Could you check a few things on this model? Use its own coordinates, in mm. Face numbers are marked on the shaded views. A direction names the side the tool comes from. Give positions to 0.01 mm unless a question says otherwise; leave off trailing zeros. Write each loop counter-clockwise with the first axis right and the second up, starting at its lowest first coordinate (ties: lowest second). Pieces come first, ordered by that corner, then holes. Notation, with made-up numbers: M 41.25,58 L 57.25,58 A17 ccw 57.25,66 Z; hole C -36.5,42 d5. An arc over 180 degrees is marked long. Answer as a JSON object with one key per item and string values. Group by question number.
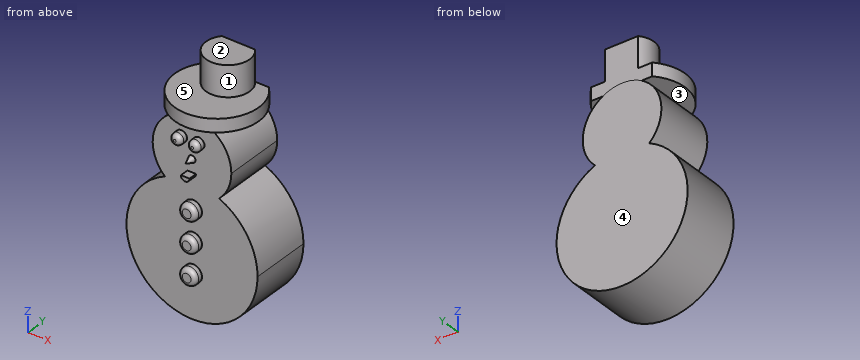
```python
from build123d import *

# Parameters (mm, degrees)
F1_DEPTH  = 7
F2_DEPTH  = 7
F3_R      = 1
F4_DEPTH  = 1
F5_DEPTH  = 1
F6_DEPTH  = 1
F7_R      = 0.65
F8_DEPTH  = 1
F9_DEPTH  = 1
F14_DEPTH = 1.5
F16_DEPTH = 3.5
F18_DEPTH = 1
F19_R     = 0.5


# Not quite as in the source:
# - a feature names something its author has since deleted; it is built from what else it names


with BuildPart() as f1:
    # F0 (on Front) → F1 (new body)
    with BuildSketch(Plane.XZ):
        with BuildLine():
            ThreePointArc((-3.1083265336, 6.8255626992), (0, 5.5795304558), (3.1083265336, 6.8255626992))
            ThreePointArc((3.1083265336, 6.8255626992), (0, 7.5), (-3.1083265336, 6.8255626992))
        make_face()
        with BuildLine():
            ThreePointArc((-3.1083265336, 6.8255626992), (0, 7.5), (3.1083265336, 6.8255626992))
            ThreePointArc((3.1083265336, 6.8255626992), (4.1374792689, 8.3099922958), (4.5, 10.0795304558))
            ThreePointArc((4.5, 10.0795304558), (-1.7695381599, 14.2170097247), (-3.1083265336, 6.8255626992))
        make_face()
    extrude(amount=F1_DEPTH)

    # F0 (on Front) → F2 (join)
    with BuildSketch(Plane.XZ):
        with BuildLine():
            ThreePointArc((-3.1083265336, 6.8255626992), (-4.0581739119, -6.3072358844), (7.5, 0))
            ThreePointArc((7.5, 0), (6.3072358844, 4.0581739119), (3.1083265336, 6.8255626992))
            ThreePointArc((3.1083265336, 6.8255626992), (0, 5.5795304558), (-3.1083265336, 6.8255626992))
        make_face()
    extrude(amount=F2_DEPTH)

    # F3 (on face) → F4 (join)
    with BuildSketch(Plane.XZ.offset(7)):
        with Locations((0.1404315871, 4.5206134686)):
            Circle(F3_R)
    extrude(amount=F4_DEPTH)

    # F3 (on face) → F5 (join)
    with BuildSketch(Plane.XZ.offset(7)):
        with Locations((0.1404315871, 1.0206134686)):
            Circle(F3_R)
    extrude(amount=F5_DEPTH)

    # F3 (on face) → F6 (join)
    with BuildSketch(Plane.XZ.offset(7)):
        with Locations((0.1404315871, -2.4793865314)):
            Circle(F3_R)
    extrude(amount=F6_DEPTH)

    # F7 (on face) → F8 (join)
    with BuildSketch(Plane.XZ.offset(7)):
        with Locations((-1.2232928476, 11.9385918571)):
            Circle(F7_R)
    extrude(amount=F8_DEPTH)

    # F7 (on face) → F9 (join)
    with BuildSketch(Plane.XZ.offset(7)):
        with Locations((0.7767071524, 11.9385918571)):
            Circle(F7_R)
    extrude(amount=F9_DEPTH)

    # F10 (on Right) → F11 (revolve)
    with BuildSketch(Plane.YZ):
        Polygon((-7.9928543597, 9.9160444998), (-6.9928543597, 9.9160444998), (-6.9928543597, 10.3160444998), align=None)
    revolve(axis=Axis((0, -7.4928543597, 9.9160444998), (0, -1, 0)))

    # F13 (on offset) → F14 (join)
    with BuildSketch(Plane.XY.offset(14)):
        with BuildLine():
            Line((3.561746113, -0.0150235719), (-3.438253887, -0.0150235719))
            ThreePointArc((-3.438253887, -0.0150235719), (0.061746113, -8.099837113), (3.561746113, -0.0150235719))
        make_face()
    extrude(amount=F14_DEPTH)

    # F15 (on face) → F16 (join)
    with BuildSketch(Plane.XY.offset(15.5)):
        with BuildLine():
            Line((1.9837659688, -0.0150235719), (-1.8346020611, -0.0150235719))
            ThreePointArc((-1.8346020611, -0.0150235719), (0.0745819538, -4.1290298907), (1.9837659688, -0.0150235719))
        make_face()
    extrude(amount=F16_DEPTH)

    # F17 (on face) → F18 (join)
    with BuildSketch(Plane.XZ.offset(7)):
        with BuildLine():
            Line((0.4505876301, 8.4716784917), (-0.5113184951, 8.4716784917))
            ThreePointArc((-0.5113184951, 8.4716784917), (-0.5247841756, 8.4659470606), (-0.5299885637, 8.4522690419))
            ThreePointArc((-0.5299885637, 8.4522690419), (-0.0303654325, 7.9716784917), (0.4692576987, 8.4522690419))
            ThreePointArc((0.4692576987, 8.4522690419), (0.4640533106, 8.4659470606), (0.4505876301, 8.4716784917))
        make_face()
    extrude(amount=F18_DEPTH)

    # F19
    f19_edges = [f1.edges().sort_by_distance(p)[0] for p in [
        (-1.873293, -8, 11.938592),
        (0.126707, -8, 11.938592),
        (-0.859568, -8, 4.520613),
        (-0.859568, -8, 1.020613),
        (-0.859568, -8, -2.479387),
    ]]
    fillet(f19_edges, radius=F19_R)


solid = f1.part
```
1) If we section it at B-B, the plane x = -5: List the corners of the cut face in (y, z) for me, plus the area to 3 significant figures.
2) I'm going to push flat-ended pins straight in: pin 1 (1.5 mm diameter, centred on y = -1.5, z = -4, fed in from +X); pin 2 (0.5 mm diameter, centred on x = 0, z = 4.5, fed in from -Y); pin 3 (4 mm diameter, centred on x = 5, y = -1.5, fed in from -Z). Where does each tip first touch, or does it pass through?
3) We'd pull the mould along Z, two halves only. Please class the marked faces 3, 4 and 5: released by +Z, released by -Z, zero draft, split by the parting line, or undercut.
4) If we section it at C-C, the plane z = -5.25: List the corners of the cut face in (x, y) for me, plus the area to 3 significant figures.
5) For the marked faces 1 and 2, which set-ups out of +Z, -Z, +X, -X, +Y, -Y let a thin tool reach every point of the face, with its end or its side?
6) If we section it at A-A, the plane y = -1.75: List the corners of the cut face in (x, z) for me, plus the area to 3 significant figures.
7) If we section it at D-D, the plane y = -6.25: List the corners of the cut face in (x, z) for me, plus the area to 3 significant figures.
8) Please list where these lines run through material, in increasing order: line 1 along Y through (x, z) = (-2.25, -2.75); line 2 along Z through (x, y) = (-3, -5.75); line 3 along Z through (x, y) = (2.75, -5). Write a range as from..to.
Taken from the geometry:
{
 "1": {"outline": "M -7,-5.59 L 0,-5.59 L 0,5.59 L -7,5.59 Z", "area": "78.3 mm²"},
 "2": {"pin 1": "x = 6.76", "pin 2": "y = -8", "pin 3": "z = -6.87"},
 "3": {"face 3": "undercut", "face 4": "zero draft", "face 5": "released by +Z"},
 "4": {"outline": "M -5.36,-7 L 5.36,-7 L 5.36,0 L -5.36,0 Z", "area": "75.0 mm²"},
 "5": {"face 1": "+Z", "face 2": "+Z, +X, -X, +Y, -Y"},
 "6": {"outline": "M -4.48,14 L -2.21,14 A4.5 ccw -3.11,6.83 A7.5 ccw long 3.11,6.83 A4.5 ccw 2.21,14 L 4.6,14 L 4.6,15.5 L 2.57,15.5 L 2.57,19 L -2.42,19 L -2.42,15.5 L -4.48,15.5 Z", "area": "262 mm²"},
 "7": {"outline": "M -3.72,14 L -2.21,14 A4.5 ccw -3.11,6.83 A7.5 ccw long 3.11,6.83 A4.5 ccw 2.21,14 L 3.85,14 L 3.85,15.5 L -3.72,15.5 Z", "area": "242 mm²"},
 "8": {"line 1": "-7..0", "line 2": "-6.87..13.43, 14..15.5", "line 3": "-6.98..13.64, 14..15.5"}
}
